Design review of the part shown in the three views and the two pictorial views. Dimensions are in mm from the part's minimum x, y and z. A direction names the side the tool comes from. Coordinates: 2 decimals unless noted, no trailing zeros. Loops run counter-clockwise (first coordinate to the right, second up) from the corner with the lowest first, then second, coordinate; pieces in that order, holes last. Notation, with made-up numbers: (-37.5, 26.25) - (-30.5, 26.25) arc R19 ccw to (-30.5, 38.25) - close; hole circle Ø11 at (20, 3.25). An arc over 180 degrees is marked (long way). One line per item, written item: value. Start each with the question number.
1. Insertion check: pin 1 (8 mm diameter, centred on x = 51, y = 8.5, fed in from +Z); pin 2 (5.5 mm diameter, centred on y = 57, z = 42, fed in from -X); pin 3 (11 mm diameter, centred on x = 16, z = 44.5, fed in from -Y); pin 4 (2 mm diameter, centred on x = 15, z = 43, fed in from +Y). Each pin has a flat end and moves straight along its axis. Give the tip position at first contact, or say it passes through.
2. Take a section at C-C, the plane z = 16. State the section outline as (x, y) points.
3. The part is to be moulded in two halves that separate along Y. For the marked faces 1, 2 and 3, say which applies: released by +Y, released by -Y, zero draft, split by the parting line, or undercut.
4. Take a section at B-B, the plane z = 43. State the section outline as (x, y) points, and give its area (3 significant figures).
5. Take a section at D-D, the plane x = 65.5. State the section outline as (y, z) points, and give its area (3 significant figures).
6. For the marked faces 4, 5 and 6, list the 3-axis set-ups (+Z, -Z, +X, -X, +Y, -Y) from which the entire face can be reached by the end or side of a thin tool; tool diameter is ignored.
7. Take a section at A-A, the plane x = 55. State the section outline as (y, z) points.
8. To check wall thickness, follow line 1 (X direction, y = 58.15, z = 43); line 2 (Y direction, x = 19, z = 12); line 3 (Z direction, x = 55.5, y = 7). State the ranges of each line that lie inside material, in increasing order. Write a range as from..to.
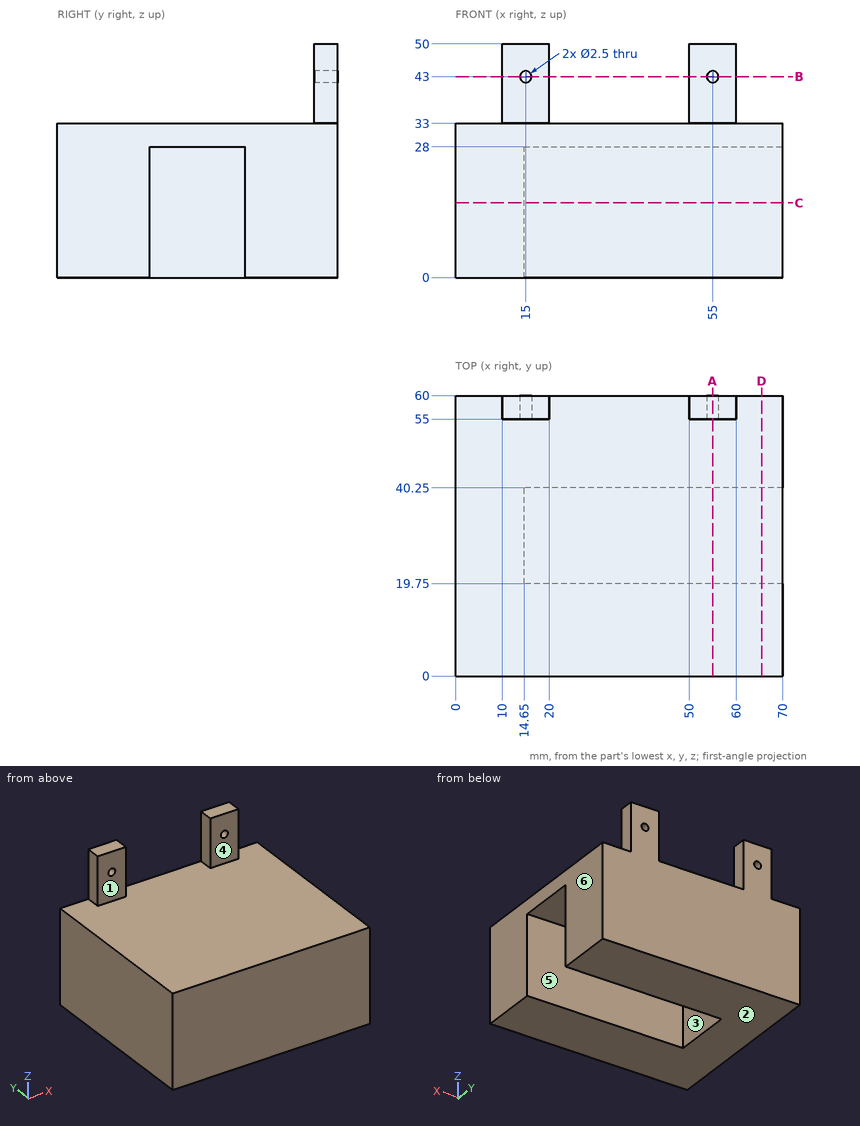
Solutions:
1. pin 1: z = 33
1. pin 2: x = 10
1. pin 3: y = 55
1. pin 4: through
2. outline: (0, 0) - (70, 0) - (70, 19.75) - (14.65, 19.75) - (14.65, 40.25) - (70, 40.25) - (70, 60) - (0, 60) - close
3. face 1: released by -Y
3. face 2: zero draft
3. face 3: undercut
4. outline: (10, 55) - (13.75, 55) - (13.75, 60) - (10, 60) - close; (16.25, 55) - (20, 55) - (20, 60) - (16.25, 60) - close; (50, 55) - (53.75, 55) - (53.75, 60) - (50, 60) - close; (56.25, 55) - (60, 55) - (60, 60) - (56.25, 60) - close
4. area: 75.0 mm2
5. outline: (0, 0) - (19.75, 0) - (19.75, 28) - (40.25, 28) - (40.25, 0) - (60, 0) - (60, 33) - (0, 33) - close
5. area: 1,410 mm2
6. face 4: +Z, +X, -X, -Y
6. face 5: -Z, +X
6. face 6: +Z, -Z, +X, +Y, -Y
7. outline: (0, 0) - (19.75, 0) - (19.75, 28) - (40.25, 28) - (40.25, 0) - (60, 0) - (60, 41.75) - (55, 41.75) - (55, 33) - (0, 33) - close; (55, 44.25) - (60, 44.25) - (60, 50) - (55, 50) - close
8. line 1: 10..13.75, 16.25..20, 50..53.75, 56.25..60
8. line 2: 0..19.75, 40.25..60
8. line 3: 0..33
